Read the model definition and answer for the solid it produces. Units are mm, in the model's axes. Face numbers are marked on the shaded views. A direction names the side the tool comes from. Give positions to 0.01 mm unless a question says otherwise; leave off trailing zeros. Loops run counter-clockwise (first coordinate to the right, second up) from the corner with the lowest first, then second, coordinate; pieces in that order, holes last. Notation, with made-up numbers: (22.5, 67.25) - (74.5, 67.25) arc R14 ccw to (74.5, 78.25) - close; hole circle Ø10 at (-14.5, 85). An arc over 180 degrees is marked (long way). Write item = value, one per line.
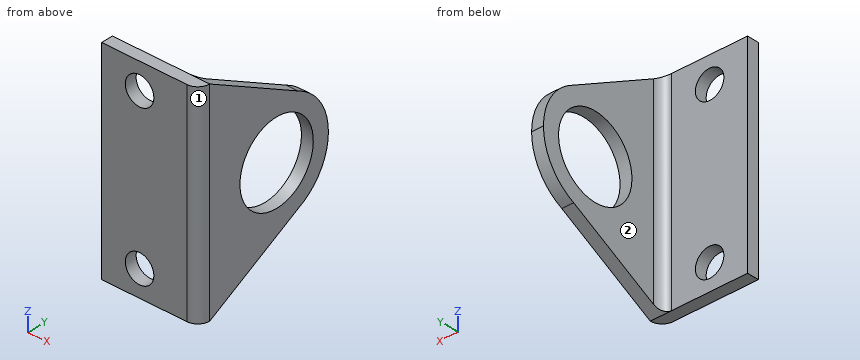
```python
from build123d import *

# Parameters (mm, degrees)
SKETCH1_W              = 18
SKETCH1_H              = 44
BOSS_EXTRUDE1_DEPTH    = 2.5
SKETCH2_R              = 3
CUT_EXTRUDE1_DEPTH     = 2.5
SKETCH3_W              = 44
SKETCH3_H              = 30
BOSS_EXTRUDE2_DEPTH    = 2.5
CUT_EXTRUDE2_START     = -2.5
CUT_EXTRUDE2_OUTLINE_R = 8.5
CUT_EXTRUDE2_DEPTH     = 2.5
FILLET7_R              = 2.5
FILLET8_R              = 2


# Read off the part's stored shape, not the designer's step: Cut-Extrude2
with BuildPart() as part:
    # Sketch1 → Boss-Extrude1 (new body)
    with BuildSketch(Plane(origin=(0, 0, 0), x_dir=(1, 0, 0), z_dir=(0, 1, 0))):
        Rectangle(SKETCH1_W, SKETCH1_H)
    extrude(amount=BOSS_EXTRUDE1_DEPTH)

    # Sketch2 → Cut-Extrude1 (cut)
    with BuildSketch(Plane(origin=(0, 2.5, 0), x_dir=(1, 0, 0), z_dir=(0, 1, 0))):
        with Locations(Location((-1, -16.5, 0), (0, 0, 270))):
            Circle(SKETCH2_R)
        with Locations(Location((-1, 16.5, 0), (0, 0, 90))):
            Circle(SKETCH2_R)
    extrude(amount=-CUT_EXTRUDE1_DEPTH, mode=Mode.SUBTRACT)

    # Sketch3 → Boss-Extrude2 (add)
    with BuildSketch(Plane(origin=(9, 0, 0), x_dir=(0, 0, -1), z_dir=(1, 0, 0))):
        with Locations((0, 15)):
            Rectangle(SKETCH3_W, SKETCH3_H)
    extrude(amount=BOSS_EXTRUDE2_DEPTH)

    # Cut-Extrude2 outline → Cut-Extrude2 (cut)
    with BuildSketch(Plane(origin=(11.5, 0, 0), x_dir=(0, 0, -1), z_dir=(1, 0, 0)).offset(CUT_EXTRUDE2_START)):
        with BuildLine():
            ThreePointArc((-10.912541818, 22.991653356), (-6.484608549, 28.09703046), (0, 30.000007173))
            Line((0, 30.000007173), (-22, 30))
            Line((-22, 30), (-22, 2.5))
            Line((-22, 2.5), (-10.912541818, 22.991653356))
        make_face()
        with BuildLine():
            ThreePointArc((0, 30.000007173), (6.484608549, 28.09703046), (10.912541818, 22.991653356))
            Line((10.912541818, 22.991653356), (22, 2.5))
            Line((22, 2.5), (22, 30))
            Line((22, 30), (0, 30.000007173))
        make_face()
        with Locations((0, 18)):
            Circle(CUT_EXTRUDE2_OUTLINE_R)
    extrude(amount=CUT_EXTRUDE2_DEPTH, mode=Mode.SUBTRACT)

    # Fillet7
    fillet7_edges = [part.edges().sort_by_distance(p)[0] for p in [
        (11.5, 0, 0),
    ]]
    fillet(fillet7_edges, radius=FILLET7_R)

    # Fillet8
    fillet8_edges = [part.edges().sort_by_distance(p)[0] for p in [
        (9, 2.5, 0),
    ]]
    fillet(fillet8_edges, radius=FILLET8_R)


solid = part.part
```
1) Each of these flat-tipped pins is pushed along its axis until it touches: P1, Ø6, axis at x = 6, y = 4, coming from the +Z side; P2, Ø5, axis at x = 3.5, z = 11.5, coming from the +Y side. Where does it stop, or does it pass through?
Output:
P1 = 22
P2 = 2.5
2) A tool of negligible diameter and unlimited length cuts with its end or side. For the marked faces 1 and 2, from which of +Z, -Z, +X, -X, +Y, -Y can it reach the whole face along a straight path? Write none if from no direction.
Output:
face_1 = +Z, -Z, +X, -Y
face_2 = +Z, -Z, -X, +Y
3) A cutting plane is placed at A-A on x = -1. Determine the outline of the cut face in (y, z).
Output:
outline = (0, -22) - (2.5, -22) - (2.5, -19.5) - (0, -19.5) - close; (0, -13.5) - (2.5, -13.5) - (2.5, 13.5) - (0, 13.5) - close; (0, 19.5) - (2.5, 19.5) - (2.5, 22) - (0, 22) - close
4) A cutting plane is placed at D-D on y = 24.5. Determine the outline of the cut face in (x, z), then the cut area to 3 significant figures.
Output:
outline = (9, -10.09) - (11.5, -10.09) - (11.5, -5.48) - (9, -5.48) - close; (9, 5.48) - (11.5, 5.48) - (11.5, 10.09) - (9, 10.09) - close
area = 23.0 mm²
5) A cutting plane is placed at B-B on z = -16.5. Determine the outline of the cut face in (x, y) (3 decimals).
Output:
outline = (-9, 0) - (-4, 0) - (-4, 2.5) - (-9, 2.5) - close; (2, 0) - (9, 0) arc R2.5 ccw to (11.5, 2.5) - (11.5, 12.665) - (9, 12.665) - (9, 4.5) arc R2 cw to (7, 2.5) - (2, 2.5) - close
6) A cutting plane is placed at C-C on y = 18. Determine the outline of the cut face in (x, z), then the cut area to 3 significant figures.
Output:
outline = (9, -13.61) - (11.5, -13.61) - (11.5, -8.5) - (9, -8.5) - close; (9, 8.5) - (11.5, 8.5) - (11.5, 13.61) - (9, 13.61) - close
area = 25.6 mm²
7) Find the intervals of material crossed by probe 1 along X at (y, z) = (1.3, -16.5); probe 2 along X at (y, z) = (6.75, 7); probe 3 along X at (y, z) = (1.9, 16.5), in increasing order.
Output:
probe_1 = -9 to -4, 2 to 11.19
probe_2 = 9 to 11.5
probe_3 = -9 to -4, 2 to 11.43
